Read the model definition and answer for the solid it produces. Units are mm, in the model's axes. A direction names the side the tool comes from. Round coordinates to 2 decimals unless told otherwise and drop trailing zeros. Write each loop counter-clockwise with the first axis right and the second up, starting at its lowest first coordinate (ties: lowest second). Pieces come first, ordered by that corner, then holes. Notation, with made-up numbers: (24, -40) - (69, -40) arc R19 cw to (69, -23) - close; hole circle Ø6 at (44.5, 83). An arc over 180 degrees is marked (long way). Use one line per item in the form item = value. Start each with the question number.
1) The part is cut by section C-C, the plane z = 37.5. Give the vertices of the cut face in (x, y), plus the area to 3 significant figures.
2) The part is cut by section A-A, the plane z = 14.5. Give the vertices of the cut face in (x, y).
3) For a pull along X with two mould halves and no side action, classify faces 1 (the face through (35.18, 14.9, 38.63)), 2 (the face through (-70, 15, -76.2)), 3 (the face through (-114.506, 14.901, 51.048)) as released by +X, released by -X, zero draft, split by the parting line, or undercut.
4) The part is cut by section B-B, the plane y = 24. Give the vertices of the cut face in (x, z), plus the area to 3 significant figures.
5) Each of these flat-tipped pins is pushed along its axis until it touches: pin 1 (1 mm diameter, centred on x = -96, y = 23, fed in from +Z); pin 2 (10 mm diameter, centred on x = -52, z = -15, fed in from -Y); pin 3 (3 mm diameter, centred on x = -34, y = 8, fed in from +Z); pin 4 (3 mm diameter, centred on x = 49.5, y = 27, fed in from +Z). Where does it stop, or does it pass through?
6) Consider line 1 along X through (y, z) = (28, 62); line 2 along X through (y, z) = (22, -68); line 3 along Z through (x, y) = (-45, 17). Determine where each line is inside the solid, lowest interval first. Write a range as from..to.
7) The part is cut by section D-D, the plane x = -26. Give the vertices of the cut face in (y, z), plus the area to 3 significant figures.
8) For faces 4 (the face through (94.794, 15, -1)), 5 (the face through (-34.211, 14.901, 37.567)), determine the directions among +Z, -Z, +X, -X, +Y, -Y from which every point of the face is accessible in a straight line to the end or side of a thin tool.
from build123d import *

# Parameters (mm, degrees)
F1_DEPTH = 30.226


with BuildPart() as f1:
    # F0 (on Front) → F1 (new body)
    with BuildSketch(Plane.XZ):
        with BuildLine():
            Line((69.394091, 76.2), (0, 0))
            Line((0, 0), (-69.394091, 76.2))
            Line((-69.394091, 76.2), (-94.794091, 76.2))
            Line((-94.794091, 76.2), (-134.777937, 25.181414))
            ThreePointArc((-134.777937, 25.181414), (-145.457577, -9.876098), (-129.769607, -42.996657))
            Line((-129.769607, -42.996657), (-94.794091, -76.2))
            Line((-94.794091, -76.2), (-43.994091, -76.2))
            ThreePointArc((-43.994091, -76.2), (0, -50.8), (43.994091, -76.2))
            Line((43.994091, -76.2), (94.794091, -76.2))
            Line((94.794091, -76.2), (94.794091, 76.2))
            Line((94.794091, 76.2), (69.394091, 76.2))
        make_face()
    extrude(amount=-F1_DEPTH)


solid = f1.part
Geometry results:
q1.outline = (-125.12, 0) - (-34.15, 0) - (-34.15, 30.23) - (-125.12, 30.23) - close; (34.15, 0) - (94.79, 0) - (94.79, 30.23) - (34.15, 30.23) - close
q1.area = 4,580 mm2
q2.outline = (-141.21, 0) - (-13.2, 0) - (-13.2, 30.23) - (-141.21, 30.23) - close; (13.2, 0) - (94.79, 0) - (94.79, 30.23) - (13.2, 30.23) - close
q3.face_1 = undercut
q3.face_2 = zero draft
q3.face_3 = released by -X
q4.outline = (-134.78, 25.18) arc R50.8 ccw to (-129.77, -43) - (-94.79, -76.2) - (-43.99, -76.2) arc R50.8 cw to (43.99, -76.2) - (94.79, -76.2) - (94.79, 76.2) - (69.39, 76.2) - (0, 0) - (-69.39, 76.2) - (-94.79, 76.2) - close
q4.area = 26,800 mm2
q5.pin_1 = 75.3
q5.pin_2 = 0
q5.pin_3 = 38.98
q5.pin_4 = 56
q6.line_1 = -105.92..-56.46, 56.46..94.79
q6.line_2 = -103.43..-38.1, 38.1..94.79
q6.line_3 = -76.2..49.41
q7.outline = (0, -57.96) - (30.23, -57.96) - (30.23, 28.55) - (0, 28.55) - close
q7.area = 2,610 mm2
q8.face_4 = +Z, -Z, +X, +Y, -Y
q8.face_5 = +Z, +Y, -Y
